The listing builds one solid part. Answer for the finished solid, in the listing's coordinates (mm). Coordinates: 2 decimals unless noted, no trailing zeros. Order: outer loops, then holes, each group sorted by start corner. A loop starts at its lowest first (then second) coordinate and runs counter-clockwise, first axis right, second up.
```python
from build123d import *

# Parameters (mm, degrees)
F0_W     = 76.2
F0_H     = 76.2
F1_DEPTH = 25.4
F2_R     = 6.35
F3_DEPTH = 76.201


with BuildPart() as f1:
    # F0 (on Top) → F1 (new body, symmetric)
    with BuildSketch(Plane.XY):
        Rectangle(F0_W, F0_H)
    extrude(amount=F1_DEPTH, both=True)

    # F2 (on face) → F3 (cut, through all)
    with BuildSketch(Plane(origin=(0, 38.1, 0), x_dir=(-1, 0, 0), z_dir=(0, 1, 0))):
        with Locations((0, 12.7)):
            Circle(F2_R)
    extrude(amount=-F3_DEPTH, mode=Mode.SUBTRACT)


solid = f1.part
```
(1) Find section C-C (y = 0.5). Write down the section's boundary in (x, z), and give its area (3 significant figures).
(2) Consider line 1 (Z direction, x = 0, y = 10.5); line 2 (X direction, y = -14.5, z = 13); line 3 (X direction, y = -6, z = 8.5). Determine where each line is inside the solid, lowest interval first.
(3) The mould has two halves that part along X. Classify faces 1 (the face through (38.1, -1, 0)), 2 (the face through (-1, -38.1, 0)), 3 (the face through (-3.414, 0.533, 18.054)), 4 (the face through (-38.1, -1, 0)): released by +X, released by -X, zero draft, split by the parting line, or undercut.
(4) Find section A-A (x = 0). Write down the section's boundary in (y, z).
(5) Find section B-B (z = 12.7). Write down the section's boundary in (x, y).
Findings below:
1. outline: (-38.1, -25.4) - (38.1, -25.4) - (38.1, 25.4) - (-38.1, 25.4) - close; hole circle Ø12.7 at (0, 12.7)
1. area: 3,740 mm2
2. line 1: z = -25.4 to 6.35, 19.05 to 25.4
2. line 2: x = -38.1 to -6.34, 6.34 to 38.1
2. line 3: x = -38.1 to -4.76, 4.76 to 38.1
3. face 1: released by +X
3. face 2: zero draft
3. face 3: undercut
3. face 4: released by -X
4. outline: (-38.1, -25.4) - (38.1, -25.4) - (38.1, 6.35) - (-38.1, 6.35) - close; (-38.1, 19.05) - (38.1, 19.05) - (38.1, 25.4) - (-38.1, 25.4) - close
5. outline: (-38.1, -38.1) - (-6.35, -38.1) - (-6.35, 38.1) - (-38.1, 38.1) - close; (6.35, -38.1) - (38.1, -38.1) - (38.1, 38.1) - (6.35, 38.1) - close
